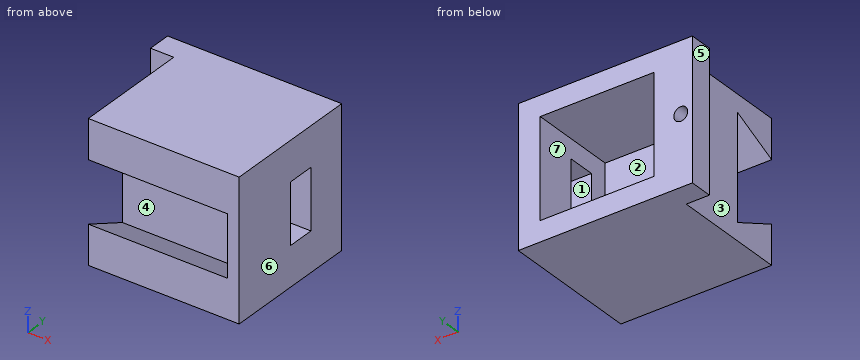
Autodesk Inventor part; units mm, degrees
ref_plane "YZ Plane" through (0, 0, 0) normal (1, 0, 0) x (0, 1, 0)
ref_plane "XZ Plane" through (0, 0, 0) normal (0, 1, 0) x (-1, 0, 0)
ref_plane "XY Plane" through (0, 0, 0) normal (0, 0, 1) x (1, 0, 0)
sketch "Sketch1" plane through (0, 0, 0) normal (1, 0, 0) x (0, 1, 0)
  line L0 (0, 0) -> (30, 0)
  line L1 (30, 0) -> (30, -30)
  line L2 (30, -30) -> (0, -30)
  line L3 (0, -30) -> (0, 0)
  line L4 (0, -8.4131) -> (10, -3.75)
  line L5 (10, -3.75) -> (10, -26.25)
  line L6 (10, -26.25) -> (0, -21.5869)
  point P0 (10, -15)
  point P1 (0, -15)
  dimension "d0" = 30
  dimension "d1" = 30
  dimension "d2" = 10
  dimension "d3" = 22.5
  dimension "d4" = 65
  dimension "d5" = 65
extrude "Extrusion1" add sketch "Sketch1" along normal blind 30 contours L0 L1 L2 L3 L6 L5 L4
sketch "Sketch2" plane through (30, 0, 0) normal (1, 0, 0) x (0, 0, -1)
  line L0 (0, 30) -> (0, 0)
  line L1 (21.5869, 0) -> (30, 0)
  line L2 (0, 30) -> (30, 30)
  line L3 (30, 30) -> (30, 0)
  line L4 (30, 0) -> (0, 0)
  line L5 (0, 0) -> (0, 30)
  point P0 (21.5869, 0)
extrude "Extrusion2" add sketch "Sketch2" along normal blind 2.5
sketch "Sketch3" plane through (0, 0, 0) normal (-1, 0, 0) x (0, 0, 1)
  line L0 (-30, 0) -> (-30, 30)
  line L1 (0, 30) -> (0, 0)
  line L2 (-30, 30) -> (0, 30)
  line L3 (0, 30) -> (0, 25)
  line L4 (0, 25) -> (-30, 25)
  line L5 (-30, 25) -> (-30, 30)
  point P0 (0, 30)
  dimension "d10" = 5
extrude "Extrusion3" add sketch "Sketch3" along normal blind 5
sketch "Sketch4" plane through (32.5, 30, 0) normal (0, 1, 0) x (1, 0, 0)
  line L0 (-32.5, 0) -> (-37.5, 0)
  line L1 (-32.5, 0) -> (-32.5, 30) construction
  circle A0 centre (-35, 15) radius 1.5
  dimension "d13" = 3
extrude "Extrusion4" cut sketch "Sketch4" against normal through all
sketch "Sketch5" plane through (32.5, 30, 0) normal (0, 1, 0) x (1, 0, 0)
  line L0 (-29.2486, 25.6211) -> (-4.7242, 25.6211)
  line L1 (-4.7242, 25.6211) -> (-4.7242, 4.3789)
  line L2 (-4.7242, 4.3789) -> (-29.2486, 4.3789)
  line L3 (-29.2486, 4.3789) -> (-29.2486, 25.6211)
  line L4 (0, 30) -> (0, 0)
  point P0 (-32.5, 0)
  point P1 (0, 15)
  point P2 (-4.7242, 15)
  point P3 (0, 15)
extrude "Extrusion5" cut sketch "Sketch5" against normal blind 19
sketch "Sketch6" plane through (32.5, 0, 0) normal (1, 0, 0) x (0, 0, -1)
  line L0 (25.6211, 11) -> (4.3789, 11)
  line L1 (8.5, 21) -> (21.5, 21)
  line L2 (21.5, 21) -> (21.5, 15)
  line L3 (21.5, 15) -> (8.5, 15)
  line L4 (8.5, 15) -> (8.5, 21)
  point P0 (0, 0)
  point P1 (15, 15)
  point P2 (15, 11)
  dimension "d18" = 13
  dimension "d19" = 6
  dimension "d20" = 4
extrude "Extrusion6" cut sketch "Sketch6" against normal up to next
properties part number "Top Sensor Mount"
Read the model definition and answer for the solid it produces. Units are mm, in the model's axes. Face numbers are marked on the shaded views. A direction names the side the tool comes from. Coordinates: 2 decimals unless noted, no trailing zeros. Order: outer loops, then holes, each group sorted by start corner. A loop starts at its lowest first (then second) coordinate and runs counter-clockwise, first axis right, second up. Notation, with made-up numbers: M 5,9 L 63,9 A27 ccw 63,25 Z; hole C -22,33 d3. An arc over 180 degrees is marked long. Put each result on its own line as item: value. Start each with the question number.
Item 1: Given pin 1 Ø1 at (x, z) = (8.5, -22) entering from +Y; pin 2 Ø1.5 at (x, z) = (-1.5, -10) entering from -Y; pin 3 Ø5 at (y, z) = (12.5, -13.5) entering from -X, each flat-ended and moving along its own axis, determine where each tip first touches the part or whether it passes through.
Item 2: Section D-D, the plane z = -21 is taken. Determine the outline of the cut face in (x, y).
Item 3: Section A-A, the plane x = -2.5 is taken. Determine the outline of the cut face in (y, z).
Item 4: Section B-B, the plane z = -14.5 is taken. Determine the outline of the cut face in (x, y), plus the area to 3 significant figures.
Item 5: For the marked faces 1, 2 and 3, determine the directions among +Z, -Z, +X, -X, +Y, -Y from which every point of the face is accessible in a straight line to the end or side of a thin tool.
Item 6: Consider probe 1 along X at (y, z) = (27.6, -15); probe 2 along Z at (x, y) = (20, 21); probe 3 along Z at (x, y) = (-2.5, 26.3). Determine where each line is inside the solid, lowest interval first. Write a range as [from, to].
Item 7: Section C-C, the plane y = 14.5 is taken. Determine the outline of the cut face in (x, z).
Item 8: The mould has two halves that part along X. Classify the marked faces 4, 5, 6 and 7: +X half, -X half, draft (parallel to the pull), parting line (faces both ways), or undercut.
Computed:
1. pin 1: stops at y = 11
1. pin 2: stops at y = 25
1. pin 3: stops at x = 0
2. outline: M -5,25 L 0,25 L 0,10 L 30,10 L 30,0 L 32.5,0 L 32.5,15 L 27.78,15 L 27.78,11 L 3.25,11 L 3.25,30 L -5,30 Z; M 27.78,21 L 32.5,21 L 32.5,30 L 27.78,30 Z
3. outline: M 25,-30 L 30,-30 L 30,-16.5 L 25,-16.5 Z; M 25,-13.5 L 30,-13.5 L 30,0 L 25,0 Z
4. outline: M -5,25 L -3.91,25 L -3.91,30 L -5,30 Z; M -1.09,25 L 0,25 L 0,10 L 30,10 L 30,0 L 32.5,0 L 32.5,15 L 27.78,15 L 27.78,11 L 3.25,11 L 3.25,30 L -1.09,30 Z; M 27.78,21 L 32.5,21 L 32.5,30 L 27.78,30 Z
4. area: 192 mm2
5. face 1: +X
5. face 2: +Y
5. face 3: +Z, -Z, -X, -Y
6. probe 1: x = [-5, -4], [-1, 3.25], [27.78, 32.5]
6. probe 2: z = [-30, -25.62], [-4.38, 0]
6. probe 3: z = [-30, -16.5], [-13.5, 0]
7. outline: M 0,-30 L 32.5,-30 L 32.5,0 L 0,0 Z; hole M 3.25,-25.62 L 27.78,-25.62 L 27.78,-4.38 L 3.25,-4.38 Z
8. face 4: draft
8. face 5: -X half
8. face 6: +X half
8. face 7: undercut
